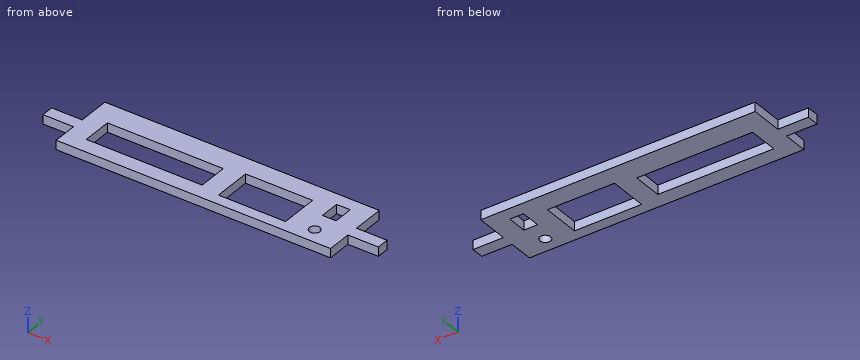
```python
from build123d import *

# Parameters (mm, degrees)
ESBO_O1_R                = 3.5
ESBO_O1_W                = 76
ESBO_O1_H                = 19.5
ESBO_O1_W_2              = 44
ESBO_O1_H_2              = 25
ESBO_O1_W_3              = 9
ESBO_O1_H_3              = 13
RESSALTO_EXTRUS_O1_DEPTH = 6


with BuildPart() as part:
    # Esboço1 → Ressalto-extrusão1 (new body)
    with BuildSketch(Plane.XY):
        Polygon((-90, -6.5), (-90, -22.5), (90, -22.5), (90, -6.5), (110, -6.5), (110, 1.5), (90, 1.5), (90, 22.5), (-90, 22.5), (-90, 1.5), (-110, 1.5), (-110, -6.5), align=None)
        with Locations((72.5, -12.5)):
            Circle(ESBO_O1_R, mode=Mode.SUBTRACT)
        with Locations((-39.333333333, -2.75)):
            Rectangle(ESBO_O1_W, ESBO_O1_H, mode=Mode.SUBTRACT)
        with Locations((33.333333333, -2.75)):
            Rectangle(ESBO_O1_W_2, ESBO_O1_H_2, mode=Mode.SUBTRACT)
        with Locations((72.5, 7.5)):
            Rectangle(ESBO_O1_W_3, ESBO_O1_H_3, mode=Mode.SUBTRACT)
    extrude(amount=RESSALTO_EXTRUS_O1_DEPTH)


solid = part.part
```
For this review, take the finished solid that the model builds, in its own axes (mm). Coordinates: 2 decimals unless noted, no trailing zeros. Order: outer loops, then holes, each group sorted by start corner. A loop starts at its lowest first (then second) coordinate and runs counter-clockwise, first axis right, second up. Notation, with made-up numbers: (85.25, 76.25) -> (143.25, 76.25) arc R16 cw to (143.25, 87.25) -> close; hole circle Ø8 at (78.5, 22.25). An arc over 180 degrees is marked (long way). Use CSV: the item, a comma, the result in double quotes. Start each with the question number.
Item 1: We need section D-D, the plane y = 18. Give the boundary of the cut face in (x, z), then the cut area to 3 significant figures.
Item 2: We need section A-A, the plane x = -17.5. Give the boundary of the cut face in (y, z), then the cut area to 3 significant figures.
Item 3: Insertion check: pin 1 (1.8 mm diameter, centred on y = 9, z = 4, fed in from +X). The pin has a flat end and moves straight along its axis. Give the tip position at first contact, or say it passes through.
Item 4: We need section C-C, the plane x = 72.5. Give the boundary of the cut face in (y, z), then the cut area to 3 significant figures.
Item 5: We need section B-B, the plane z = 2.1. Give the boundary of the cut face in (x, y).
Item 6: Wall thickness on probe 1 along X at (y, z) = (8, 5.7); probe 2 along X at (y, z) = (-2, 0.95); probe 3 along X at (y, z) = (6.5, 3.9): over which ranges is each line inside the solid? List them lowest first.
Derived:
1,outline,"(-90, 0) -> (90, 0) -> (90, 6) -> (-90, 6) -> close"
1,area,"1,080 mm^2"
2,outline,"(-22.5, 0) -> (-12.5, 0) -> (-12.5, 6) -> (-22.5, 6) -> close; (7, 0) -> (22.5, 0) -> (22.5, 6) -> (7, 6) -> close"
2,area,"153 mm^2"
3,pin 1,"stops at x = 90"
4,outline,"(-22.5, 0) -> (-16, 0) -> (-16, 6) -> (-22.5, 6) -> close; (-9, 0) -> (1, 0) -> (1, 6) -> (-9, 6) -> close; (14, 0) -> (22.5, 0) -> (22.5, 6) -> (14, 6) -> close"
4,area,"150 mm^2"
5,outline,"(-110, -6.5) -> (-90, -6.5) -> (-90, -22.5) -> (90, -22.5) -> (90, -6.5) -> (110, -6.5) -> (110, 1.5) -> (90, 1.5) -> (90, 22.5) -> (-90, 22.5) -> (-90, 1.5) -> (-110, 1.5) -> close; hole (-77.33, -12.5) -> (-1.33, -12.5) -> (-1.33, 7) -> (-77.33, 7) -> close; hole (11.33, -15.25) -> (55.33, -15.25) -> (55.33, 9.75) -> (11.33, 9.75) -> close; hole (68, 1) -> (77, 1) -> (77, 14) -> (68, 14) -> close; hole circle Ø7 at (72.5, -12.5)"
6,probe 1,"x = -90 to 11.33, 55.33 to 68, 77 to 90"
6,probe 2,"x = -110 to -77.33, -1.33 to 11.33, 55.33 to 110"
6,probe 3,"x = -90 to -77.33, -1.33 to 11.33, 55.33 to 68, 77 to 90"
